Autodesk Inventor part; units mm, degrees
ref_plane "YZ Plane" through (0, 0, 0) normal (1, 0, 0) x (0, 1, 0)
ref_plane "XZ Plane" through (0, 0, 0) normal (0, 1, 0) x (-1, 0, 0)
ref_plane "XY Plane" through (0, 0, 0) normal (0, 0, 1) x (1, 0, 0)
sketch "スケッチ1" plane through (0, 0, 0) normal (0, 0, 1) x (1, 0, 0)
  circle A0 centre (233.68, 2.54) radius 2.25 construction
  circle A1 centre (161.29, 2.54) radius 2.25 construction
  circle A2 centre (29.21, 2.54) radius 2.25 construction
  circle A3 centre (233.68, 160.02) radius 2.25 construction
  circle A4 centre (161.29, 160.02) radius 2.25 construction
  circle A5 centre (6.35, 160.02) radius 2.25 construction
  circle A6 centre (6.35, 284.48) radius 2.25 construction
  circle A7 centre (161.29, 284.48) radius 2.25 construction
  circle A8 centre (233.68, 284.48) radius 2.25 construction
  circle A9 centre (29.21, 2.54) radius 1.6
  circle A10 centre (161.29, 2.54) radius 1.6
  circle A11 centre (233.68, 2.54) radius 1.6
  circle A12 centre (233.68, 160.02) radius 1.6
  circle A13 centre (161.29, 160.02) radius 1.6
  circle A14 centre (6.35, 160.02) radius 1.6
  circle A15 centre (6.35, 284.48) radius 1.6
  circle A16 centre (161.29, 284.48) radius 1.6
  circle A17 centre (233.68, 284.48) radius 1.6
  line L0 (495.19, -98.01) -> (-14.81, -98.01)
  line L1 (-14.81, -98.01) -> (-14.81, 311.99)
  line L2 (-14.81, 311.99) -> (495.19, 311.99)
  line L3 (495.19, 311.99) -> (495.19, -98.01)
  line L4 (490.19, 306.99) -> (-9.81, 306.99) construction
  line L5 (-9.81, 306.99) -> (-9.81, -93.01) construction
  line L6 (-9.81, -93.01) -> (490.19, -93.01) construction
  line L7 (490.19, -93.01) -> (490.19, 306.99) construction
  circle A18 centre (-9.81, 306.99) radius 2.1
  circle A19 centre (490.19, 306.99) radius 2.1
  circle A20 centre (490.19, -93.01) radius 2.1
  circle A21 centre (-9.81, -93.01) radius 2.1
  circle A22 centre (-9.81, 6.99) radius 2.1
  circle A23 centre (-9.81, 106.99) radius 2.1
  circle A24 centre (-9.81, 206.99) radius 2.1
  circle A25 centre (90.19, 306.99) radius 2.1
  circle A26 centre (190.19, 306.99) radius 2.1
  circle A27 centre (290.19, 306.99) radius 2.1
  circle A28 centre (390.19, 306.99) radius 2.1
  line L8 (490.19, 106.99) -> (-9.81, 106.99) construction
  line L9 (240.19, -93.01) -> (240.19, 306.99) construction
  circle A29 centre (90.19, -93.01) radius 2.1
  circle A30 centre (190.19, -93.01) radius 2.1
  circle A31 centre (290.19, -93.01) radius 2.1
  circle A32 centre (390.19, -93.01) radius 2.1
  circle A33 centre (490.19, 6.99) radius 2.1
  circle A34 centre (490.19, 106.99) radius 2.1
  circle A35 centre (490.19, 206.99) radius 2.1
  point P0 (0, 0)
  point P1 (-3.81, 297.18)
  point P2 (0, 300.99)
  point P3 (3.7629, -59.9187)
  point P4 (-9.81, 106.99)
  dimension "d0" = 3.2
  dimension "d1" = 510
  dimension "d2" = 410
  dimension "d3" = 11
  dimension "d4" = 11
  dimension "d5" = 5
  dimension "d6" = 4.2
  dimension "d7" = 4.2
  dimension "d8" = 4.2
  dimension "d9" = 4.2
  dimension "d10" = 100
  dimension "d11" = 100
  dimension "d13" = 100
  dimension "d14" = 100
  dimension "d15" = 100
  dimension "d16" = 100
  dimension "d17" = 100
  dimension "d18" = 100
  dimension "d19" = 100
  dimension "d23" = 4.2
  dimension "d24" = 4.2
  dimension "d25" = 4.2
  dimension "d26" = 100
  dimension "d27" = 100
  dimension "d55" = 100
extrude "押し出し1" add sketch "スケッチ1" along normal blind 3
fillet "フィレット1" radius 5 4 edges at (495.19, -98.01, 1.5) (-14.81, -98.01, 1.5) (-14.81, 311.99, 1.5) (495.19, 311.99, 1.5)
sketch "スケッチ2" plane through (0, 0, 3) normal (0, 0, 1) x (1, 0, 0)
  line L0 (-6.934, 160.0686) -> (-6.134, 160.0686) construction
  line L1 (-6.134, 160.0686) -> (-6.134, 170.6186) construction
  line L2 (-6.134, 170.6186) -> (-6.934, 170.6186) construction
  line L3 (-6.934, 170.6186) -> (-6.934, 160.0686) construction
  line L4 (-6.934, 159.9686) -> (-6.134, 159.9686) construction
  line L5 (-6.134, 170.7186) -> (-6.934, 170.7186)
  arc A0 (-7.334, 161.353) -> (-6.934, 159.9686) centre (-6.934, 160.7186) ccw
  line L6 (-5.734, 159.9686) -> (-5.734, 170.7186) construction
  arc A1 (-6.934, 170.7186) -> (-7.334, 169.3342) centre (-6.934, 169.9686) ccw
  line L7 (-7.334, 161.353) -> (-7.334, 169.3342)
  arc A2 (-6.134, 159.9686) -> (-6.134, 161.4686) centre (-6.134, 160.7186) ccw construction
  arc A3 (-6.134, 169.2186) -> (-6.134, 170.7186) centre (-6.134, 169.9686) ccw construction
  arc A4 (-6.134, 159.9686) -> (-5.734, 161.353) centre (-6.134, 160.7186) ccw
  arc A5 (-5.734, 169.3342) -> (-6.134, 170.7186) centre (-6.134, 169.9686) ccw
  line L8 (-5.734, 161.353) -> (-5.734, 169.3342)
  line L9 (-6.934, 159.9686) -> (-6.134, 159.9686)
  line L10 (-7.334, 181.753) -> (-7.334, 189.7342)
  arc A6 (-7.334, 181.753) -> (-6.934, 180.3686) centre (-6.934, 181.1186) ccw
  arc A7 (-6.134, 180.3686) -> (-5.734, 181.753) centre (-6.134, 181.1186) ccw
  line L11 (-5.734, 181.753) -> (-5.734, 189.7342)
  line L12 (-6.934, 180.3686) -> (-6.134, 180.3686)
  arc A8 (-6.934, 191.1186) -> (-7.334, 189.7342) centre (-6.934, 190.3686) ccw
  line L13 (-6.134, 191.1186) -> (-6.934, 191.1186)
  arc A9 (-5.734, 189.7342) -> (-6.134, 191.1186) centre (-6.134, 190.3686) ccw
  line L14 (-7.334, 202.153) -> (-7.334, 210.1342)
  arc A10 (-7.334, 202.153) -> (-6.934, 200.7686) centre (-6.934, 201.5186) ccw
  arc A11 (-6.134, 200.7686) -> (-5.734, 202.153) centre (-6.134, 201.5186) ccw
  line L15 (-5.734, 202.153) -> (-5.734, 210.1342)
  line L16 (-6.934, 200.7686) -> (-6.134, 200.7686)
  arc A12 (-6.934, 211.5186) -> (-7.334, 210.1342) centre (-6.934, 210.7686) ccw
  line L17 (-6.134, 211.5186) -> (-6.934, 211.5186)
  arc A13 (-5.734, 210.1342) -> (-6.134, 211.5186) centre (-6.134, 210.7686) ccw
  line L18 (-7.334, 222.553) -> (-7.334, 230.5342)
  arc A14 (-7.334, 222.553) -> (-6.934, 221.1686) centre (-6.934, 221.9186) ccw
  arc A15 (-6.134, 221.1686) -> (-5.734, 222.553) centre (-6.134, 221.9186) ccw
  line L19 (-5.734, 222.553) -> (-5.734, 230.5342)
  line L20 (-6.934, 221.1686) -> (-6.134, 221.1686)
  arc A16 (-6.934, 231.9186) -> (-7.334, 230.5342) centre (-6.934, 231.1686) ccw
  line L21 (-6.134, 231.9186) -> (-6.934, 231.9186)
  arc A17 (-5.734, 230.5342) -> (-6.134, 231.9186) centre (-6.134, 231.1686) ccw
  line L22 (-7.334, 242.953) -> (-7.334, 250.9342)
  arc A18 (-7.334, 242.953) -> (-6.934, 241.5686) centre (-6.934, 242.3186) ccw
  arc A19 (-6.134, 241.5686) -> (-5.734, 242.953) centre (-6.134, 242.3186) ccw
  line L23 (-5.734, 242.953) -> (-5.734, 250.9342)
  line L24 (-6.934, 241.5686) -> (-6.134, 241.5686)
  arc A20 (-6.934, 252.3186) -> (-7.334, 250.9342) centre (-6.934, 251.5686) ccw
  line L25 (-6.134, 252.3186) -> (-6.934, 252.3186)
  arc A21 (-5.734, 250.9342) -> (-6.134, 252.3186) centre (-6.134, 251.5686) ccw
  line L26 (-7.334, 263.353) -> (-7.334, 271.3342)
  arc A22 (-7.334, 263.353) -> (-6.934, 261.9686) centre (-6.934, 262.7186) ccw
  arc A23 (-6.134, 261.9686) -> (-5.734, 263.353) centre (-6.134, 262.7186) ccw
  line L27 (-5.734, 263.353) -> (-5.734, 271.3342)
  line L28 (-6.934, 261.9686) -> (-6.134, 261.9686)
  arc A24 (-6.934, 272.7186) -> (-7.334, 271.3342) centre (-6.934, 271.9686) ccw
  line L29 (-6.134, 272.7186) -> (-6.934, 272.7186)
  arc A25 (-5.734, 271.3342) -> (-6.134, 272.7186) centre (-6.134, 271.9686) ccw
  line L30 (-7.334, 283.753) -> (-7.334, 291.7342)
  arc A26 (-7.334, 283.753) -> (-6.934, 282.3686) centre (-6.934, 283.1186) ccw
  arc A27 (-6.134, 282.3686) -> (-5.734, 283.753) centre (-6.134, 283.1186) ccw
  line L31 (-5.734, 283.753) -> (-5.734, 291.7342)
  line L32 (-6.934, 282.3686) -> (-6.134, 282.3686)
  arc A28 (-6.934, 293.1186) -> (-7.334, 291.7342) centre (-6.934, 292.3686) ccw
  line L33 (-6.134, 293.1186) -> (-6.934, 293.1186)
  arc A29 (-5.734, 291.7342) -> (-6.134, 293.1186) centre (-6.134, 292.3686) ccw
  point P0 (0, 0)
  point P1 (-6.934, 180.4686)
  point P2 (-6.134, 191.0186)
  dimension "d34" = 20.4
  dimension "d37" = 1.5
  dimension "d39" = 0.1
  dimension "d40" = 0.1
  dimension "d41" = 1.6
  dimension "d42" = 0.8
  dimension "d43" = 0.4
  dimension "d46" = 20.4
extrude "押し出し2" [suppressed]
sketch "スケッチ6" plane through (0, 0, 3) normal (0, 0, 1) x (1, 0, 0)
  arc A0 (379.99, -128.01) -> (100.39, -128.01) centre (240.19, -438.744) ccw
  arc A1 (483.7257, -128.01) -> (483.7257, 341.99) centre (-161.4767, 106.99) ccw
  arc A2 (79.99, 341.99) -> (400.39, 341.99) centre (240.19, 754.724) ccw
  arc A3 (-3.3457, 341.99) -> (-3.3457, -128.01) centre (641.8567, 106.99) ccw
  line L0 (-9.81, -98.01) -> (490.19, -98.01)
  arc A4 (490.19, -98.01) -> (495.19, -93.01) centre (490.19, -93.01) ccw
  line L1 (495.19, -93.01) -> (495.19, 306.99)
  arc A5 (495.19, 306.99) -> (490.19, 311.99) centre (490.19, 306.99) ccw
  line L2 (490.19, 311.99) -> (-9.81, 311.99)
  arc A6 (-9.81, 311.99) -> (-14.81, 306.99) centre (-9.81, 306.99) ccw
  line L3 (-14.81, 306.99) -> (-14.81, -93.01)
  arc A7 (-14.81, -93.01) -> (-9.81, -98.01) centre (-9.81, -93.01) ccw
  line L4 (483.7257, -128.01) -> (379.99, -128.01)
  line L5 (100.39, -128.01) -> (-3.3457, -128.01)
  line L6 (483.7257, 341.99) -> (400.39, 341.99)
  line L7 (79.99, 341.99) -> (-3.3457, 341.99)
  point P0 (0, 0)
  point P1 (-14.59, 308.457)
  point P2 (-14.59, -94.477)
  point P3 (494.97, -94.477)
  point P4 (494.97, 308.457)
  point P5 (240.19, 311.99)
  point P6 (240.19, -98.01)
extrude "押し出し5" add sketch "スケッチ6" against normal up to surface (3 mm away) contours A5 L2 A2 L6 A1 | A3 L7 A2 L2 A6
sketch "スケッチ7" plane through (0, 0, 3) normal (0, 0, 1) x (1, 0, 0)
  arc A0 (495.19, 306.99) -> (494.97, 308.457) centre (490.19, 306.99) ccw
  arc A1 (494.97, 308.457) -> (483.7257, 341.99) centre (-161.4767, 106.99) ccw
  arc A2 (-3.3457, 341.99) -> (-14.59, 308.457) centre (641.8567, 106.99) ccw
  arc A3 (-14.59, 308.457) -> (-14.81, 306.99) centre (-9.81, 306.99) ccw
  line L0 (-14.81, 306.99) -> (-14.81, 336.99)
  line L1 (-9.81, 341.99) -> (-3.3457, 341.99)
  arc A4 (495.19, 306.99) -> (494.97, 308.457) centre (490.19, 306.99) ccw
  line L2 (495.19, 306.99) -> (495.19, 336.99)
  line L3 (483.7257, 341.99) -> (400.39, 341.99)
  line L4 (490.19, 341.99) -> (483.7257, 341.99)
  arc A5 (-9.81, 341.99) -> (-14.81, 336.99) centre (-9.81, 336.99) ccw
  arc A6 (495.19, 336.99) -> (490.19, 341.99) centre (490.19, 336.99) ccw
  point P0 (0, 0)
  point P1 (-14.81, 341.99)
  point P2 (495.19, 341.99)
  dimension "d62" = 5
extrude "押し出し6" add sketch "スケッチ7" against normal up to surface (3 mm away)
fillet "フィレット2" radius 5 2 edges at (400.39, 341.99, 1.5) (79.99, 341.99, 1.5)
sketch "スケッチ8" plane through (0, 0, 3) normal (0, 0, 1) x (1, 0, 0)
  circle A0 centre (490.19, -93.01) radius 2.1 construction
  circle A1 centre (-9.81, -93.01) radius 2.1 construction
  arc A2 (-9.81, 341.99) -> (-14.81, 336.99) centre (-9.81, 336.99) ccw construction
  arc A3 (495.19, 336.99) -> (490.19, 341.99) centre (490.19, 336.99) ccw construction
  circle A4 centre (479.19, -82.01) radius 2.1
  circle A5 centre (1.19, -82.01) radius 2.1
  circle A6 centre (1.19, 325.99) radius 2.1
  circle A7 centre (479.19, 325.99) radius 2.1
  circle A8 centre (490.19, 336.99) radius 2.1
  circle A9 centre (-9.81, 336.99) radius 2.1
  arc A10 (401.3236, 341.99) -> (399.5242, 341.655) centre (401.3236, 336.99) ccw construction
  arc A11 (80.8558, 341.655) -> (79.0564, 341.99) centre (79.0564, 336.99) ccw construction
  circle A12 centre (79.0564, 336.99) radius 2.1
  circle A13 centre (401.3236, 336.99) radius 2.1
  point P0 (0, 0)
  dimension "d63" = 11
  dimension "d64" = 11
  dimension "d65" = 11
  dimension "d66" = 11
  dimension "d67" = 11
  dimension "d68" = 11
  dimension "d69" = 11
  dimension "d70" = 11
extrude "押し出し7" cut sketch "スケッチ8" against normal through all
sketch "スケッチ9" plane through (0, 0, 0) normal (0, 0, -1) x (-1, 0, 0)
  circle A0 centre (-490.19, 6.99) radius 2.1 construction
  line L0 (-490.19, 6.99) -> (-490.19, -23.01) construction
  circle A1 centre (-490.19, -23.01) radius 2.1
  circle A2 centre (-490.19, 106.99) radius 2.1 construction
  line L1 (-490.19, 106.99) -> (-490.19, 136.99) construction
  circle A3 centre (-490.19, 136.99) radius 2.1
  circle A4 centre (9.81, 206.99) radius 2.1 construction
  line L2 (9.81, 206.99) -> (9.81, 176.99) construction
  circle A5 centre (9.81, 176.99) radius 2.1
  circle A6 centre (-490.19, 121.99) radius 2.1
  circle A7 centre (9.81, 191.99) radius 2.1
  circle A8 centre (9.81, 161.99) radius 2.1
  circle A9 centre (9.81, 306.99) radius 2.1 construction
  circle A10 centre (9.81, 336.99) radius 2.1 construction
  circle A11 centre (9.81, 336.99) radius 2.1 construction
  line L3 (9.81, 306.99) -> (9.81, 336.99) construction
  circle A12 centre (9.81, 321.99) radius 2.1
  circle A13 centre (-490.19, -8.01) radius 2.1
  circle A14 centre (9.81, 6.99) radius 2.1 construction
  line L4 (9.81, 6.99) -> (9.81, -23.01) construction
  circle A15 centre (9.81, -23.01) radius 2.1
  point P0 (0, 0)
  dimension "d74" = 30
  dimension "d77" = 15
  dimension "d78" = 30
extrude "押し出し8" cut sketch "スケッチ9" against normal through all
equation "\"d10\" = -0.5 * d5 + 0.25 * d2"
equation "\"d11\" = d10"
equation "\"d13\" = -0.4 * d5 + 0.2 * d1"
equation "\"d14\" = d13"
equation "\"d15\" = d13"
equation "\"d16\" = d13"
equation "\"d17\" = d20"
equation "\"d18\" = d20"
equation "\"d19\" = d20"
equation "\"d26\" = d28"
equation "\"d27\" = d26"
equation "\"d40\" = d39"
equation "\"d43\" = -0.5 * d42 + 0.5 * d41"
equation "\"d46\" = d34"
equation "\"d65\" = d63"
equation "\"d66\" = d63"
equation "\"d67\" = d63"
equation "\"d68\" = d63"
equation "\"d69\" = d63"
equation "\"d70\" = d63"
equation "\"d77\" = 0.5 * d74"
equation "\"d20\" = -0.4 * d22 + 0.2 * d21"
equation "\"d28\" = -0.5 * d30 + 0.25 * d29"
properties part number "riglt_plate_01"
For this review, take the finished solid that the model builds, in its own axes (mm). Round coordinates to 2 decimals unless told otherwise and drop trailing zeros. Order: outer loops, then holes, each group sorted by start corner. A loop starts at its lowest first (then second) coordinate and runs counter-clockwise, first axis right, second up. Notation, with made-up numbers: (-36, 33.5) -> (5, 33.5) arc R12 cw to (5, 49.5) -> close; hole circle Ø5 at (26, 2.5). An arc over 180 degrees is marked (long way). Put each result on its own line as item: value.
Q1. Mouldability with a two-part tool opening along X and no side actions: class faces 1 (the flat face through (237, 125, 3)), 2 (the cylindrical face through (237.908, 311.996, 1.521)) as pulls with the +X half, pulls with the -X half, needs draft (parallel to the pull), parting line crosses it, or undercut.
Check result:
face 1: needs draft
face 2: undercut
Q2. Add section B-B on x = 257.5. Write out the cut boundary in (y, z).
Check result:
outline: (-98.01, 0) -> (312.33, 0) -> (312.33, 3) -> (-98.01, 3) -> close
Q3. Add section C-C on x = 348.5. Write out the cut boundary in (y, z), plus the area to 3 significant figures.
Check result:
outline: (-98.01, 0) -> (325.44, 0) -> (325.44, 3) -> (-98.01, 3) -> close
area: 1,270 mm2
Q4. Add section A-A on z = 0.45. State how many separate pieces and enclosed holes the cut face has, plus the area to 3 significant figures.
Check result:
separate pieces: 1
enclosed holes: 44
area: 217,000 mm2
Q5. For probe 1 along X at (y, z) = (192.5, 2.2); probe 2 along X at (y, z) = (284.48, 1.1); probe 3 along X at (y, z) = (191.99, 1.05), list the stretches that pass through material, from the lowest coordinate up. Write a range as [from, to].
Check result:
probe 1: [-14.81, -11.85], [-7.77, 495.19]
probe 2: [-14.81, 4.75], [7.95, 159.69], [162.89, 232.08], [235.28, 495.19]
probe 3: [-14.81, -11.91], [-7.71, 495.19]
Q6. Insertion check: pin 1 Ø5 at (x, y) = (161.29, 284.48) entering from +Z; pin 2 Ø2.5 at (x, y) = (-9.81, -23.01) entering from -Z. Each pin has a flat end and moves straight along its axis. Give the tip position at first contact, or say it passes through.
Check result:
pin 1: z = 3
pin 2: through
